Work out the finished part from the listing and answer in its coordinate system (mm). A direction names the side the tool comes from. Round coordinates to 2 decimals unless told otherwise and drop trailing zeros. Order: outer loops, then holes, each group sorted by start corner. A loop starts at its lowest first (then second) coordinate and runs counter-clockwise, first axis right, second up. Notation, with made-up numbers: M -30,-33 L -14,-33 A20 cw -14,-26 Z; hole C -39,52.25 d7. An arc over 180 degrees is marked long. Return JSON: item names as keys, results as strings.
from build123d import *

# Parameters (mm, degrees)
F1_DEPTH = 25.4
F3_DEPTH = 25.4


# Not quite as in the source:
# - a feature names something its author has since deleted; it is built from what else it names


with BuildPart() as f1:
    # F0 (on Top) → F1 (new body)
    with BuildSketch(Plane.XY):
        Polygon((-27.94, 43.9866697311), (-53.755334568, 43.9866697311), (-53.755334568, -32.2133302689), (22.444665432, -32.2133302689), (22.444665432, 43.9866697311), (0, 43.9866697311), (0, 5.8866697311), (-27.94, 5.8866697311), align=None)
    extrude(amount=F1_DEPTH)

    # F2 (on face) → F3 (cut)
    with BuildSketch(Plane.XY.offset(25.4)):
        Polygon((-27.94, 43.9866697311), (-31.5155684948, 43.9866697311), (-31.5155684948, 0), (-31.5155684948, -10.3501314297), (0, -10.3501314297), (0, 5.8866697311), (-27.94, 5.8866697311), align=None)
    extrude(amount=-F3_DEPTH, mode=Mode.SUBTRACT)


solid = f1.part
Item 1: Which of the six approach directions +Z, -Z, +X, -X, +Y, -Y give full straight-line access (tool end or side, diameter ignored) to faces 1 (the flat face through (-42, 43.987, 13)), 2 (the flat face through (0, 16, 13))?
Output:
{"face 1": "+Z, -Z, +X, -X, +Y", "face 2": "+Z, -Z, +Y"}
Item 2: Find section B-B (z = 20.75). Determine the outline of the cut face in (x, y), plus the area to 3 significant figures.
Output:
{"outline": "M -53.76,-32.21 L 22.44,-32.21 L 22.44,43.99 L 0,43.99 L 0,-10.35 L -31.52,-10.35 L -31.52,43.99 L -53.76,43.99 Z", "area": "4,090 mm^2"}
Item 3: Find section C-C (x = -4). Determine the outline of the cut face in (y, z), plus the area to 3 significant figures.
Output:
{"outline": "M -32.21,0 L -10.35,0 L -10.35,25.4 L -32.21,25.4 Z", "area": "555 mm^2"}
Item 4: This flat-tipped pin is pushed along its axis until it touches: pin 1 (7.5 mm diameter, centred on x = -22.5, z = 17, fed in from +Y). Where does it stop, or does it pass through?
Output:
{"pin 1": "stops at y = -10.35"}
Item 5: Consider line 1 along X through (y, z) = (11, 12.75); line 2 along Y through (x, z) = (-30, 9.5). Determine where each line is inside the solid, lowest interval first. Write a range as [from, to].
Output:
{"line 1": "x = [-53.76, -31.52], [0, 22.44]", "line 2": "y = [-32.21, -10.35]"}
Item 6: Find section A-A (y = 5). Determine the outline of the cut face in (x, z), plus the area to 3 significant figures.
Output:
{"outline": "M -53.76,0 L -31.52,0 L -31.52,25.4 L -53.76,25.4 Z; M 0,0 L 22.44,0 L 22.44,25.4 L 0,25.4 Z", "area": "1,130 mm^2"}
Item 7: The mould has two halves that part along X. Classify faces 3 (the flat face through (-16, -11, 25.4)), 4 (the flat face through (22.445, 5, 13)), 5 (the flat face through (-16, -10.35, 13)), 6 (the flat face through (-31.516, 17, 13)): pulls with the +X half, pulls with the -X half, needs draft (parallel to the pull), parting line crosses it, or undercut.
Output:
{"face 3": "needs draft", "face 4": "pulls with the +X half", "face 5": "undercut", "face 6": "undercut"}
